from build123d import *

# Parameters (mm, degrees)
BOSS_EXTRUDE1_DEPTH          = 152.4
BOSS_EXTRUDE1_DEPTH_BACK     = 152.4
SKETCH3_W                    = 304.8
SKETCH3_H                    = 1.5875
SKETCH4_W                    = 304.8
SKETCH4_H                    = 304.8
CUT_EXTRUDE1_DEPTH           = 2.54
F_10_0_1935_DIAMETER_HOLE1_D = 4.9149
CIRPATTERN1_START            = -0.79375
CIRPATTERN1_OUTLINE_R        = 2.45745
CIRPATTERN1_DEPTH            = 1.5875


# Read off the part's stored shape, not the designer's step: CirPattern1
with BuildPart() as part:
    # Sketch3 → Boss-Extrude1 (new, two sides: drawn at the far end of the back side and taken through both)
    with BuildSketch(Plane.XY.offset(-BOSS_EXTRUDE1_DEPTH_BACK)):
        Rectangle(SKETCH3_W, SKETCH3_H)
    extrude(amount=BOSS_EXTRUDE1_DEPTH + BOSS_EXTRUDE1_DEPTH_BACK)

    # Sketch4 → Cut-Extrude1 (cut)
    # profile 1 of 2: a face of its own
    with BuildSketch(Plane(origin=(0, 0.79375, 0), x_dir=(1, 0, 0), z_dir=(0, 1, 0))):
        Rectangle(SKETCH4_W, SKETCH4_H)
        with BuildLine():
            Line((15.875, -45.57424684), (15.875, -72.579138876))
            ThreePointArc((15.875, -72.579138876), (-74.295, 0), (15.875, 72.579138876))
            Line((15.875, 72.579138876), (15.875, 45.57424684))
            ThreePointArc((15.875, 45.57424684), (-48.26, 0), (15.875, -45.57424684))
        make_face(mode=Mode.SUBTRACT)
    # profile 2 of 2: a face of its own
    with BuildSketch(Plane(origin=(0, 0.79375, 0), x_dir=(1, 0, 0), z_dir=(0, 1, 0))):
        with BuildLine():
            Line((-6.35, 60.628368772), (-6.35, 70.835950618))
            ThreePointArc((-6.35, 70.835950618), (-71.12, 0), (-6.35, -70.835950618))
            Line((-6.35, -70.835950618), (-6.35, -60.628368772))
            ThreePointArc((-6.35, -60.628368772), (-60.96, 0), (-6.35, 60.628368772))
        make_face()
    extrude(amount=-CUT_EXTRUDE1_DEPTH, mode=Mode.SUBTRACT)

    # #10 (0.1935) Diameter Hole1 (through all)
    with Locations(Plane(origin=(-53.975, 0.79375, 0), x_dir=(0, 0, 1), z_dir=(0, 1, 0))):
        with Locations((0, 0)):
            Hole(F_10_0_1935_DIAMETER_HOLE1_D / 2)

    # CirPattern1 outline → CirPattern1 (cut)
    with BuildSketch(Plane(origin=(0, 0, 0), x_dir=(1, 0, 0), z_dir=(0, 1, 0)).offset(CIRPATTERN1_START)):
        with Locations((-44.21373159, 30.958788152)):
            Circle(CIRPATTERN1_OUTLINE_R)
        with Locations((-18.460537236, 50.719909207)):
            Circle(CIRPATTERN1_OUTLINE_R)
        with BuildLine():
            Line((15.875, 50.583714627), (15.875, 53.687978321))
            ThreePointArc((15.875, 53.687978321), (11.512307959, 52.135846474), (15.875, 50.583714627))
        make_face()
        with Locations((-44.21373159, -30.958788152)):
            Circle(CIRPATTERN1_OUTLINE_R)
        with Locations((-18.460537236, -50.719909207)):
            Circle(CIRPATTERN1_OUTLINE_R)
    extrude(amount=CIRPATTERN1_DEPTH, mode=Mode.SUBTRACT)


solid = part.part
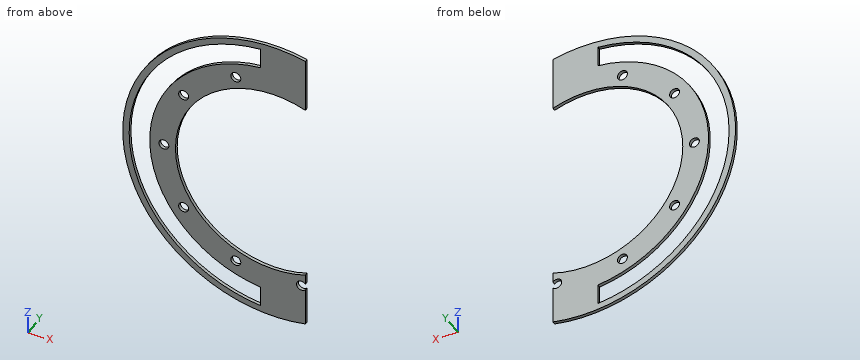
The listing builds one solid part. Answer for the finished solid, in the listing's coordinates (mm). Round coordinates to 2 decimals unless told otherwise and drop trailing zeros. Order: outer loops, then holes, each group sorted by start corner. A loop starts at its lowest first (then second) coordinate and runs counter-clockwise, first axis right, second up. Notation, with made-up numbers: (81.5, 89) -> (92.5, 89) arc R20 ccw to (92.5, 117) -> close; hole circle Ø5 at (-26.5, 71). An arc over 180 degrees is marked (long way). Put each result on its own line as item: value.
Q1. Each of these flat-tipped pins is pushed along its axis until it touches: P1, Ø8, axis at x = -18.46, z = 50.72, coming from the -Y side; P2, Ø0.5, axis at y = 0, z = 67.5, coming from the -X side. Where does it stop, or does it pass through?
Results list:
P1: y = -0.79
P2: x = -31.58
Q2. Section A-A, the plane x = 0 is taken. Write down the section's boundary in (y, z) (3 decimals), and give its area (3 significant figures).
Results list:
outline: (-0.794, -74.295) -> (0.794, -74.295) -> (0.794, -48.26) -> (-0.794, -48.26) -> close; (-0.794, 48.26) -> (0.794, 48.26) -> (0.794, 74.295) -> (-0.794, 74.295) -> close
area: 82.7 mm^2
Q3. Section B-B, the plane z = 0 is taken. Write down the section's boundary in (x, y) (3 decimals).
Results list:
outline: (-74.295, -0.794) -> (-71.12, -0.794) -> (-71.12, 0.794) -> (-74.295, 0.794) -> close; (-60.96, -0.794) -> (-56.432, -0.794) -> (-56.432, 0.794) -> (-60.96, 0.794) -> close; (-51.518, -0.794) -> (-48.26, -0.794) -> (-48.26, 0.794) -> (-51.518, 0.794) -> close
Q4. Section D-D, the plane y = 0.05 is taken. Write down the section's boundary in (x, z) (3 decimals), and give its area (3 significant figures).
Results list:
outline: (15.875, -72.579) -> (15.875, -53.688) arc R2.457 cw (long way) to (15.875, -50.584) -> (15.875, -45.574) arc R48.26 cw (long way) to (15.875, 45.574) -> (15.875, 72.579) arc R74.295 ccw (long way) to start; hole circle Ø4.915 at (-53.975, 0); hole circle Ø4.915 at (-44.214, -30.959); hole circle Ø4.915 at (-44.214, 30.959); hole circle Ø4.915 at (-18.461, -50.72); hole circle Ø4.915 at (-18.461, 50.72); hole (-6.35, -70.836) -> (-6.35, -60.628) arc R60.96 cw to (-6.35, 60.628) -> (-6.35, 70.836) arc R71.12 ccw to start
area: 3,760 mm^2
Q5. Section C-C, the plane x = -13.5 is taken. Write down the section's boundary in (y, z).
Results list:
outline: (-0.79, -73.06) -> (0.79, -73.06) -> (0.79, -69.83) -> (-0.79, -69.83) -> close; (-0.79, -59.45) -> (0.79, -59.45) -> (0.79, -46.33) -> (-0.79, -46.33) -> close; (-0.79, 46.33) -> (0.79, 46.33) -> (0.79, 59.45) -> (-0.79, 59.45) -> close; (-0.79, 69.83) -> (0.79, 69.83) -> (0.79, 73.06) -> (-0.79, 73.06) -> close
Q6. Consider line 1 along X through (y, z) = (-0.7, 49.5) (3 decimals); line 2 along Z through (x, y) = (1, -0.1); line 3 along Z through (x, y) = (-55, 0.65). Determine where each line is inside the solid, lowest interval first.
Results list:
line 1: -55.403 to -51.067, -35.579 to -20.594, -16.327 to 15.875
line 2: -74.29 to -48.25, 48.25 to 74.29
line 3: -49.95 to -45.09, -26.29 to -2.23, 2.23 to 26.29, 45.09 to 49.95
